CAD build for the part. Positions are in the model's coordinates, mm. A direction names the side the tool comes from. Coordinates: 2 decimals unless noted, no trailing zeros. Loops run counter-clockwise (first coordinate to the right, second up) from the corner with the lowest first, then second, coordinate; pieces in that order, holes last. Notation, with made-up numbers: (-20, -9.75) -> (12, -9.75) arc R15 cw to (12, 2.25) -> close; hole circle Ø11 at (72, -2.5). An arc over 180 degrees is marked (long way). Write each question's results on one line, items separated by ' | '.
```python
from build123d import *

# Parameters (mm, degrees)
BOSS_EXTRUDE1_DEPTH            = 7.5
BOSS_EXTRUDE1_DEPTH_BACK       = 7.5
CUT_EXTRUDE3_REACH             = 31.568
SKETCH5_R                      = 1.5
FILLET1_R                      = 5
CUT_EXTRUDE2_REACH             = 19.405
SKETCH3_R                      = 1
CUT_EXTRUDE2_DIRECTION_2_REACH = 19.405
FILLET2_R                      = 5
BOSS_EXTRUDE2_START            = 3.8
SKETCH6_R                      = 1.2
BOSS_EXTRUDE2_DEPTH            = 3.7
BOSS_EXTRUDE3_START            = -7.5
SKETCH6_4_R                    = 1.2
BOSS_EXTRUDE3_DEPTH            = 3.7


with BuildPart() as part:
    # Sketch1 → Boss-Extrude1 (new, two sides: drawn at the far end of the back side and taken through both)
    with BuildSketch(Plane(origin=(0, 0, 0), x_dir=(-1, 0, 0), z_dir=(0, 1, 0)).offset(-BOSS_EXTRUDE1_DEPTH_BACK)):
        with BuildLine():
            Line((6.3, 7.5), (-6.3, 7.5))
            Line((-6.3, 7.5), (-12.102943725, 1.697056275))
            ThreePointArc((-12.102943725, 1.697056275), (-11.582689122, -0.918440238), (-13.8, -2.4))
            Line((-13.8, -2.4), (-13.8, -7.5))
            Line((-13.8, -7.5), (13.8, -7.5))
            Line((13.8, -7.5), (13.8, -2.4))
            ThreePointArc((13.8, -2.4), (11.582689122, -0.918440238), (12.102943725, 1.697056275))
            Line((12.102943725, 1.697056275), (6.3, 7.5))
        make_face()
    extrude(amount=BOSS_EXTRUDE1_DEPTH + BOSS_EXTRUDE1_DEPTH_BACK)

    # Sketch5 → Cut-Extrude3 (cut, up to next)
    with BuildSketch(Plane.YZ.offset(13.8), mode=Mode.PRIVATE) as cut_extrude3_sk1:
        with Locations(Location((-2.25, -4.95, 0), (0, 0, 270))):
            Circle(SKETCH5_R)
    cut_extrude3_tool1 = extrude(cut_extrude3_sk1.sketch, amount=-CUT_EXTRUDE3_REACH, mode=Mode.PRIVATE) & part.part
    # Sketch5 → Cut-Extrude3 (cut, up to next)
    with BuildSketch(Plane.YZ.offset(13.8), mode=Mode.PRIVATE) as cut_extrude3_sk2:
        with Locations(Location((2.25, -4.95, 0), (0, 0, 270))):
            Circle(SKETCH5_R)
    cut_extrude3_tool2 = extrude(cut_extrude3_sk2.sketch, amount=-CUT_EXTRUDE3_REACH, mode=Mode.PRIVATE) & part.part
    add(cut_extrude3_tool1.solids().sort_by_distance((13.8, -2.25, -4.95))[0], mode=Mode.SUBTRACT)
    add(cut_extrude3_tool2.solids().sort_by_distance((13.8, 2.25, -4.95))[0], mode=Mode.SUBTRACT)

    # Fillet1
    fillet1_edges = [part.edges().sort_by_distance(p)[0] for p in [
        (0, -7.5, -7.5),
        (0, 7.5, -7.5),
    ]]
    fillet(fillet1_edges, radius=FILLET1_R)

    # Cut-Extrude2: up to this plane
    cut_extrude2_end = Plane(origin=(-6.9, -7.5, 6.9), z_dir=(0.7071067811865475, 0, -0.7071067811865477))
    # Sketch3 → Cut-Extrude2 (cut, up to the surface)
    with BuildSketch(Plane.YZ, mode=Mode.PRIVATE) as cut_extrude2_sk1:
        with Locations(Location((0, 4.598528137, 0), (0, 0, 90))):
            Circle(SKETCH3_R)
    cut_extrude2_tool1 = split(extrude(cut_extrude2_sk1.sketch, amount=-CUT_EXTRUDE2_REACH, mode=Mode.PRIVATE), bisect_by=cut_extrude2_end, keep=Keep.BOTH, mode=Mode.PRIVATE)
    add(cut_extrude2_tool1.solids().sort_by_distance((0, 0, 4.598528))[0], mode=Mode.SUBTRACT)

    # Cut-Extrude2 direction 2: up to this plane
    cut_extrude2_direction_2_end = Plane(origin=(6.9, -7.5, 6.9), z_dir=(-0.7071067811865475, 0, -0.7071067811865476))
    # Sketch3 → Cut-Extrude2 direction 2 (cut, up to the surface)
    with BuildSketch(Plane.YZ, mode=Mode.PRIVATE) as cut_extrude2_direction_2_sk1:
        with Locations(Location((0, 4.598528137, 0), (0, 0, 90))):
            Circle(SKETCH3_R)
    cut_extrude2_direction_2_tool1 = split(extrude(cut_extrude2_direction_2_sk1.sketch, amount=CUT_EXTRUDE2_DIRECTION_2_REACH, mode=Mode.PRIVATE), bisect_by=cut_extrude2_direction_2_end, keep=Keep.BOTH, mode=Mode.PRIVATE)
    add(cut_extrude2_direction_2_tool1.solids().sort_by_distance((0, 0, 4.598528))[0], mode=Mode.SUBTRACT)

    # Fillet2
    fillet2_edges = [part.edges().sort_by_distance(p)[0] for p in [
        (0, 7.5, 7.5),
        (0, -7.5, 7.5),
    ]]
    fillet(fillet2_edges, radius=FILLET2_R)

    # Sketch6 → Boss-Extrude2 (add)
    # profile 1 of 2: a face of its own
    with BuildSketch(Plane(origin=(0, 0, 0), x_dir=(-1, 0, 0), z_dir=(0, 1, 0)).offset(BOSS_EXTRUDE2_START)):
        with BuildLine():
            Line((-12.102943725, 1.697056275), (-12.244365081, 1.555634919))
            ThreePointArc((-12.244365081, 1.555634919), (-15.832534972, 0.841903551), (-13.8, -2.2))
            Line((-13.8, -2.2), (-13.8, -2.4))
            ThreePointArc((-13.8, -2.4), (-11.582689122, -0.918440238), (-12.102943725, 1.697056275))
        make_face()
        with Locations(Location((-13.8, 0, 0), (0, 0, 90))):
            Circle(SKETCH6_R, mode=Mode.SUBTRACT)
    # profile 2 of 2: a face of its own
    with BuildSketch(Plane(origin=(0, 0, 0), x_dir=(-1, 0, 0), z_dir=(0, 1, 0)).offset(BOSS_EXTRUDE2_START)):
        with BuildLine():
            Line((13.8, -2.4), (13.8, -2.2))
            ThreePointArc((13.8, -2.2), (15.832534972, 0.841903551), (12.244365081, 1.555634919))
            Line((12.244365081, 1.555634919), (12.102943725, 1.697056275))
            ThreePointArc((12.102943725, 1.697056275), (11.582689122, -0.918440238), (13.8, -2.4))
        make_face()
        with Locations(Location((13.8, 0, 0), (0, 0, 270))):
            Circle(SKETCH6_R, mode=Mode.SUBTRACT)
    extrude(amount=BOSS_EXTRUDE2_DEPTH)

    # Sketch6<4> → Boss-Extrude3 (add)
    # profile 1 of 2: a face of its own
    with BuildSketch(Plane(origin=(0, 0, 0), x_dir=(-1, 0, 0), z_dir=(0, 1, 0)).offset(BOSS_EXTRUDE3_START)):
        with BuildLine():
            Line((-12.102943725, 1.697056275), (-12.244365081, 1.555634919))
            ThreePointArc((-12.244365081, 1.555634919), (-15.832534972, 0.841903551), (-13.8, -2.2))
            Line((-13.8, -2.2), (-13.8, -2.4))
            ThreePointArc((-13.8, -2.4), (-11.582689122, -0.918440238), (-12.102943725, 1.697056275))
        make_face()
        with Locations(Location((-13.8, 0, 0), (0, 0, 90))):
            Circle(SKETCH6_4_R, mode=Mode.SUBTRACT)
    # profile 2 of 2: a face of its own
    with BuildSketch(Plane(origin=(0, 0, 0), x_dir=(-1, 0, 0), z_dir=(0, 1, 0)).offset(BOSS_EXTRUDE3_START)):
        with BuildLine():
            Line((13.8, -2.4), (13.8, -2.2))
            ThreePointArc((13.8, -2.2), (15.832534972, 0.841903551), (12.244365081, 1.555634919))
            Line((12.244365081, 1.555634919), (12.102943725, 1.697056275))
            ThreePointArc((12.102943725, 1.697056275), (11.582689122, -0.918440238), (13.8, -2.4))
        make_face()
        with Locations(Location((13.8, 0, 0), (0, 0, 270))):
            Circle(SKETCH6_4_R, mode=Mode.SUBTRACT)
    extrude(amount=BOSS_EXTRUDE3_DEPTH)


solid = part.part
```
Q1. Drop flat-ended pins along their axis: pin 1 (3 mm diameter, centred on x = 13.8, z = 0, fed in from -Y); pin 2 (1.5 mm diameter, centred on y = -0.5, z = -4, fed in from +X); pin 3 (1.8 mm diameter, centred on y = 0, z = 4.6, fed in from -X); pin 4 (5 mm diameter, centred on x = 10, y = 2, fed in from +Z). Give the stop position or say it passes through.
Results are:
pin 1: y = -7.5 | pin 2: x = 13.8 | pin 3: through | pin 4: z = 6.3
Q2. Cut at B-B on y = 5.5. Write the cut outline in (x, z).
Results are:
outline: (-13.8, -6.5) -> (13.8, -6.5) -> (13.8, -2.2) arc R2.2 ccw (long way) to (12.24, 1.56) -> (7.3, 6.5) -> (-7.3, 6.5) -> (-12.24, 1.56) arc R2.2 ccw (long way) to (-13.8, -2.2) -> close; hole circle Ø2.4 at (-13.8, 0); hole circle Ø2.4 at (13.8, 0)
Q3. Cut at A-A on z = 0. Write the cut outline in (x, y).
Results are:
outline: (-16, -7.5) -> (-15, -7.5) -> (-15, -3.8) -> (-16, -3.8) -> close; (-16, 3.8) -> (-15, 3.8) -> (-15, 7.5) -> (-16, 7.5) -> close; (-12.6, -7.5) -> (12.6, -7.5) -> (12.6, -3.8) -> (11.4, -3.8) -> (11.4, 3.8) -> (12.6, 3.8) -> (12.6, 7.5) -> (-12.6, 7.5) -> (-12.6, 3.8) -> (-11.4, 3.8) -> (-11.4, -3.8) -> (-12.6, -3.8) -> close; (15, -7.5) -> (16, -7.5) -> (16, -3.8) -> (15, -3.8) -> close; (15, 3.8) -> (16, 3.8) -> (16, 7.5) -> (15, 7.5) -> close
Q4. Cut at D-D on z = 4.5. Write the cut outline in (x, y).
Results are:
outline: (-9.3, -7.08) -> (9.3, -7.08) -> (9.3, -1) -> (-9.3, -1) -> close; (-9.3, 1) -> (9.3, 1) -> (9.3, 7.08) -> (-9.3, 7.08) -> close
Q5. Which spindle directions (+Z, -Z, +X, -X, +Y, -Y) get a long thin tool onto all of the face, cutting with end or side? Do faces 1 (the cylindrical face through (15, -6, 0)), 2 (the cylindrical face through (-11.598, -0.053, -0.955)). Say none if no direction does.
Results are:
face 1: +Y, -Y | face 2: -X
Q6. Pull direction Y, two halves, no side cores. Call faces 3 (the flat face through (0, 0, 7.5)), 4 (the cylindrical face through (-0.19, -6.07, -6)), 5 (the flat face through (0, 7.5, 0)), 6 (the flat face through (12.7, 3.8, -1.1)): +Y half, -Y half, draft (parallel to the pull), parting line (faces both ways), or undercut.
Results are:
face 3: draft | face 4: -Y half | face 5: +Y half | face 6: undercut
Q7. Wall check: L1, parallel to X at y = -5.8, z = 0; L2, parallel to Y at x = -2.5, z = -5.75; L3, parallel to Y at x = 5.5, z = -4.5. Give the ranges that are in metal, low to high. Write a range as from..to.
Results are:
L1: -16..-15, -12.6..12.6, 15..16 | L2: -6.3..-3.52, -0.98..0.98, 3.52..6.3 | L3: -7.08..-3.68, -0.82..0.82, 3.68..7.08
Q8. Cut at C-C on y = 0. Write the cut outline in (x, z), and give its area (3 significant figures).
Results are:
outline: (-13.8, -7.5) -> (13.8, -7.5) -> (13.8, -2.4) arc R2.4 cw to (12.1, 1.7) -> (10.2, 3.6) -> (-10.2, 3.6) -> (-12.1, 1.7) arc R2.4 cw to (-13.8, -2.4) -> close; (-8.2, 5.6) -> (8.2, 5.6) -> (6.3, 7.5) -> (-6.3, 7.5) -> close | area: 307 mm^2
